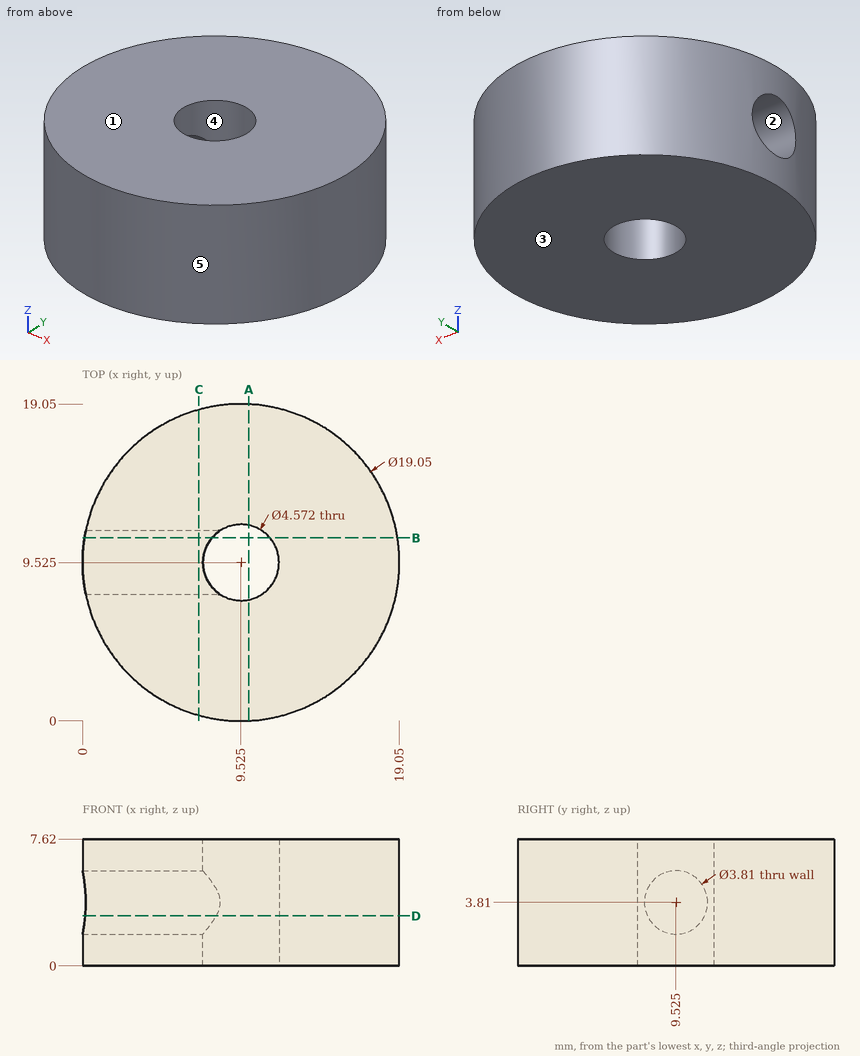
Drawing for the job (mm, zero at the part's lowest x, y, z). A direction names the side the tool comes from. Coordinates: 2 decimals unless noted, no trailing zeros. Loops run counter-clockwise (first coordinate to the right, second up) from the corner with the lowest first, then second, coordinate; pieces in that order, holes last. Notation, with made-up numbers: (3, 58.5) - (39, 58.5) arc R14 cw to (39, 78.5) - close; hole circle Ø10 at (24.25, 84). An arc over 180 degrees is marked (long way). Use CSV: the item, a comma, the result in double quotes. Start each with the question number.
Q1. Cut at D-D, the plane z = 3. List the corners of the cut face in (x, y) (3 decimals).
Q2. Cut at A-A, the plane x = 10. List the corners of the cut face in (y, z).
Q3. Cut at B-B, the plane y = 11. List the corners of the cut face in (x, z).
Q4. Probe probe 1 along Y at (x, z) = (9.5, 5.25); probe 2 along Y at (x, z) = (5, 3.75); probe 3 along X at (y, z) = (9.5, 3.75). List the from-to ranges inside material, lowest first. Write a range as from..to.
Q5. 3-axis set-ups, long thin cutter, end or side, ignore diameter. For the marked faces 1 and 2: which of +Z, -Z, +X, -X, +Y, -Y reach the whole face in a straight line?
Q6. Cut at C-C, the plane x = 7. List the corners of the cut face in (y, z) (3 decimals), then the cut area to 3 significant figures.
Q7. Drop flat-ended pins along their axis: P1, Ø4, axis at y = 8, z = 2.5, coming from the -X side; P2, Ø2, axis at y = 14, z = 3.5, coming from the -X side; P3, Ø2, axis at x = 6, z = 4.5, coming from the +Y side; P4, Ø1, axis at x = 17, y = 2.5, coming from the -Z side. Give the stop position or say it passes through.
Q8. Two-plate mould, pull along Y, no slides. Class the marked faces 3, 4 and 5: +Y half, -Y half, draft (parallel to the pull), parting line (faces both ways), or undercut.
Here are the results:
1,outline,"(0.157, 7.801) arc R9.525 ccw (long way) to (0.157, 11.249) - (8.024, 11.249) arc R2.286 cw (long way) to (8.024, 7.801) - close"
2,outline,"(0.01, 0) - (7.29, 0) - (7.29, 7.62) - (0.01, 7.62) - close; (11.76, 0) - (19.04, 0) - (19.04, 7.62) - (11.76, 7.62) - close"
3,outline,"(0.11, 0) - (7.78, 0) - (7.78, 2.6) - (0.11, 2.6) - close; (0.11, 5.02) - (7.78, 5.02) - (7.78, 7.62) - (0.11, 7.62) - close; (11.27, 0) - (18.94, 0) - (18.94, 7.62) - (11.27, 7.62) - close"
4,probe 1,"0..7.24, 11.81..19.05"
4,probe 2,"1.14..7.62, 11.43..17.91"
4,probe 3,"11.81..19.05"
5,face 1,"+Z, +X, -X, +Y, -Y"
5,face 2,"-X"
6,outline,"(0.341, 0) - (18.709, 0) - (18.709, 7.62) - (0.341, 7.62) - close; hole circle Ø3.81 at (9.525, 3.81)"
6,area,"129 mm2"
7,P1,"x = 0"
7,P2,"x = 0.66"
7,P3,"y = 18.71"
7,P4,"through"
8,face 3,"draft"
8,face 4,"undercut"
8,face 5,"parting line"
